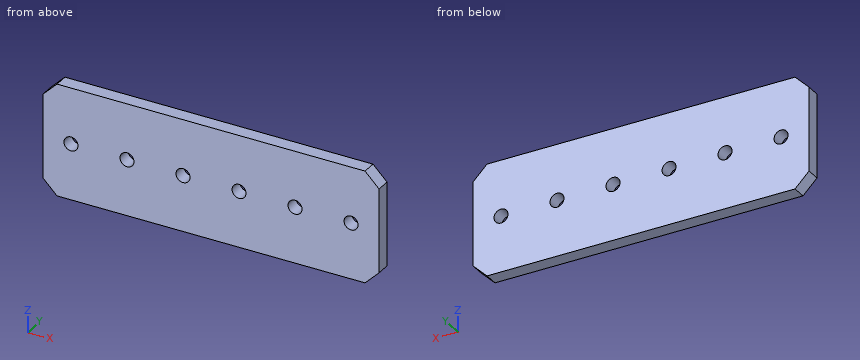
Autodesk Inventor part; units mm, degrees
ref_plane "YZ Plane" through (0, 0, 0) normal (1, 0, 0) x (0, 1, 0)
ref_plane "XZ Plane" through (0, 0, 0) normal (0, 1, 0) x (-1, 0, 0)
ref_plane "XY Plane" through (0, 0, 0) normal (0, 0, 1) x (1, 0, 0)
sketch "Sketch1" plane through (0, 0, 0) normal (0, 1, 0) x (-1, 0, 0)
  line L0 (0, 0) -> (11.2251, 0)
  circle A0 centre (6.35, -12.7) radius 1.5875
  circle A1 centre (19.05, -12.7) radius 1.5875
  circle A2 centre (31.75, -12.7) radius 1.5875
  circle A3 centre (44.45, -12.7) radius 1.5875
  circle A4 centre (57.15, -12.7) radius 1.5875
  circle A5 centre (69.85, -12.7) radius 1.5875
  line L1 (0, 0) -> (0, -22.225)
  line L2 (3.175, -25.4) -> (73.025, -25.4)
  line L3 (76.2, -22.225) -> (76.2, -3.175)
  line L4 (73.025, 0) -> (11.2251, 0)
  line L5 (73.025, 0) -> (76.2, -3.175)
  line L6 (76.2, -22.225) -> (73.025, -25.4)
  line L7 (3.175, -25.4) -> (0, -22.225)
  line L8 (3.175, 0) -> (0, -3.175)
  point P0 (5.6126, 0)
  point P1 (0, -25.4)
  point P2 (76.2, -25.4)
  point P3 (76.2, 0)
  dimension "d0" = 3.175
  dimension "d2" = 12.7
  dimension "d5" = 12.7
  dimension "d10" = 25.4
  dimension "d11" = 6.35
  dimension "d12" = 3.175
  dimension "d13" = 3.175
  dimension "d14" = 3.175
  dimension "d15" = 3.175
  dimension "d16" = 3.175
  dimension "d17" = 3.175
extrude "Extrusion1" add sketch "Sketch1" along normal blind 3.175 contours L0 L4 L5 L3 L6 L2 L7 L1 L8
properties part number "Straight Bracket (6)"
The listing builds one solid part. Answer for the finished solid, in the listing's coordinates (mm). Give positions to 0.01 mm unless a question says otherwise; leave off trailing zeros. Write each loop counter-clockwise with the first axis right and the second up, starting at its lowest first coordinate (ties: lowest second). Pieces come first, ordered by that corner, then holes. Notation, with made-up numbers: (51.5, -7.75) -> (72.5, -7.75) arc R18 ccw to (72.5, 24.25) -> close; hole circle Ø7 at (20, 54.25). An arc over 180 degrees is marked (long way). One line per question, with ' | ' between items. Start each with the question number.
1. Given pin 1 Ø5 at (x, z) = (-44.45, -12.7) entering from +Y (3 decimals); pin 2 Ø1.9 at (x, z) = (-19.05, -12.7) entering from -Y, each flat-ended and moving along its own axis, determine where each tip first touches the part or whether it passes through.
2. Section C-C (y = 1.95) is taken. State how many separate pieces and enclosed holes the cut face has, plus the area to 3 significant figures.
3. Find the intervals of material crossed by probe 1 along Z at (x, y) = (-19.05, 2.45); probe 2 along X at (y, z) = (0.9, -23.5) (3 decimals), in increasing order.
4. Section A-A (z = -12.7) is taken. Determine the outline of the cut face in (x, y) (1 decimal), plus the area to 3 significant figures.
5. Section D-D (z = -23.75) is taken. Determine the outline of the cut face in (x, y) (3 decimals).
6. Section B-B (x = -19.05) is taken. Determine the outline of the cut face in (y, z) (1 decimal).
Response values:
1) pin 1: y = 3.175 | pin 2: through
2) separate pieces: 1 | enclosed holes: 6 | area: 1,870 mm2
3) probe 1: -25.4 to -14.29, -11.11 to 0 | probe 2: -74.925 to -1.275
4) outline: (-76.2, 0) -> (-71.4, 0) -> (-71.4, 3.2) -> (-76.2, 3.2) -> close; (-68.3, 0) -> (-58.7, 0) -> (-58.7, 3.2) -> (-68.3, 3.2) -> close; (-55.6, 0) -> (-46, 0) -> (-46, 3.2) -> (-55.6, 3.2) -> close; (-42.9, 0) -> (-33.3, 0) -> (-33.3, 3.2) -> (-42.9, 3.2) -> close; (-30.2, 0) -> (-20.6, 0) -> (-20.6, 3.2) -> (-30.2, 3.2) -> close; (-17.5, 0) -> (-7.9, 0) -> (-7.9, 3.2) -> (-17.5, 3.2) -> close; (-4.8, 0) -> (0, 0) -> (0, 3.2) -> (-4.8, 3.2) -> close | area: 181 mm2
5) outline: (-74.675, 0) -> (-1.525, 0) -> (-1.525, 3.175) -> (-74.675, 3.175) -> close
6) outline: (0, -25.4) -> (3.2, -25.4) -> (3.2, -14.3) -> (0, -14.3) -> close; (0, -11.1) -> (3.2, -11.1) -> (3.2, 0) -> (0, 0) -> close
